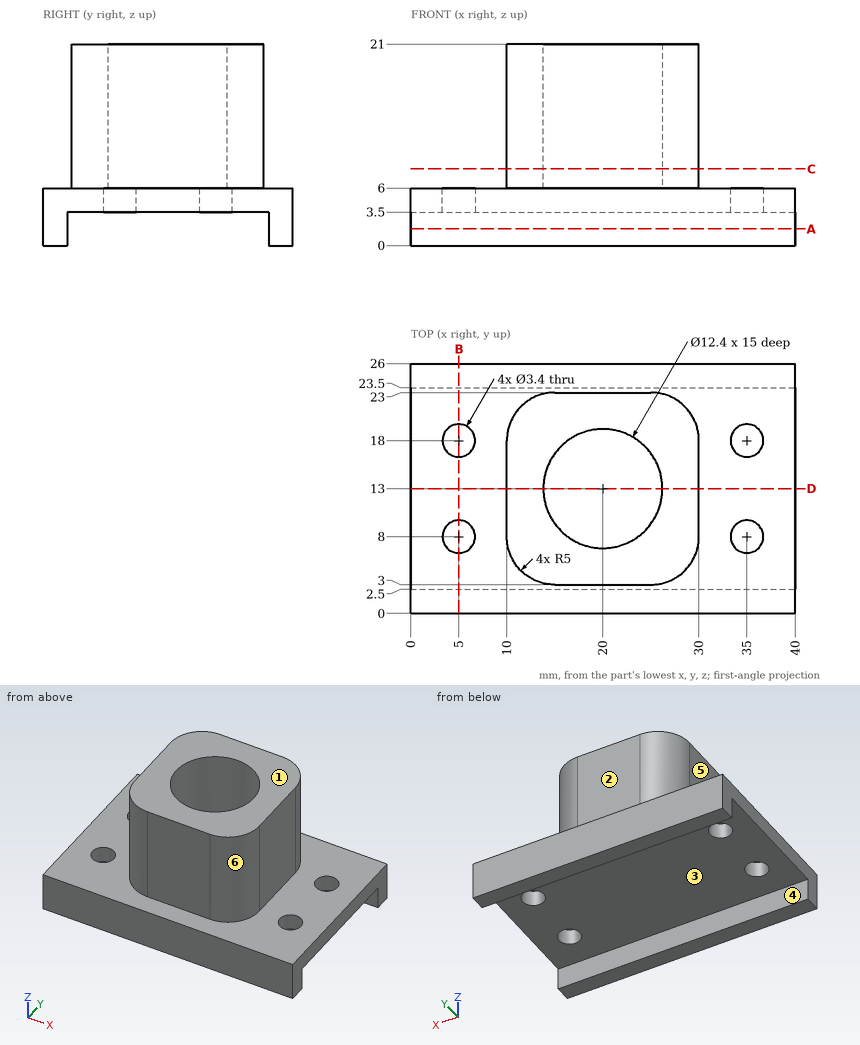
The drawing under review shows one solid part. Ordinate dimensions are in mm from its lowest x, y, z. A direction names the side the tool comes from. Round coordinates to 2 decimals unless told otherwise and drop trailing zeros. Loops run counter-clockwise (first coordinate to the right, second up) from the corner with the lowest first, then second, coordinate; pieces in that order, holes last. Notation, with made-up numbers: (28, 22) -> (58, 22) arc R23 ccw to (58, 52) -> close; hole circle Ø11 at (38, 7.25). An arc over 180 degrees is marked (long way). Answer in a Markdown table with one row per item.
1) For pin 1 Ø4.5 at (x, y) = (5, 18) entering from +Z; pin 2 Ø5.5 at (x, y) = (35, 18) entering from -Z; pin 3 Ø5 at (x, z) = (17.5, 10) entering from -Y, all flat-tipped, find the tip position at first contact; note any pin that passes through.
Taken from the geometry:
| item | result |
|---|---|
| pin 1 | stops at z = 6 |
| pin 2 | stops at z = 3.5 |
| pin 3 | stops at y = 3 |
2) Wall thickness on line 1 along Y through (x, z) = (35, 4.65); line 2 along X through (y, z) = (19, 5); line 3 along Z through (x, y) = (34.5, 6): over which ranges is each line inside the solid? List them lowest first.
Taken from the geometry:
| item | result |
|---|---|
| line 1 | y = 0 to 6.3, 9.7 to 16.3, 19.7 to 26 |
| line 2 | x = 0 to 3.63, 6.37 to 33.63, 36.37 to 40 |
| line 3 | z = 3.5 to 6 |
3) Consider section B-B, the plane x = 5. Write out the cut boundary in (y, z).
Taken from the geometry:
| item | result |
|---|---|
| outline | (0, 0) -> (2.5, 0) -> (2.5, 3.5) -> (6.3, 3.5) -> (6.3, 6) -> (0, 6) -> close; (9.7, 3.5) -> (16.3, 3.5) -> (16.3, 6) -> (9.7, 6) -> close; (19.7, 3.5) -> (23.5, 3.5) -> (23.5, 0) -> (26, 0) -> (26, 6) -> (19.7, 6) -> close |
4) Consider section D-D, the plane y = 13. Write out the cut boundary in (x, z).
Taken from the geometry:
| item | result |
|---|---|
| outline | (0, 3.5) -> (40, 3.5) -> (40, 6) -> (30, 6) -> (30, 21) -> (26.2, 21) -> (26.2, 6) -> (13.8, 6) -> (13.8, 21) -> (10, 21) -> (10, 6) -> (0, 6) -> close |
5) Consider section A-A, the plane z = 1.75. Write out the cut boundary in (x, y).
Taken from the geometry:
| item | result |
|---|---|
| outline | (0, 0) -> (40, 0) -> (40, 2.5) -> (0, 2.5) -> close; (0, 23.5) -> (40, 23.5) -> (40, 26) -> (0, 26) -> close |
6) Consider section C-C, the plane z = 8. Write out the cut boundary in (x, y), plus the area to 3 significant figures.
Taken from the geometry:
| item | result |
|---|---|
| outline | (10, 8) arc R5 ccw to (15, 3) -> (25, 3) arc R5 ccw to (30, 8) -> (30, 18) arc R5 ccw to (25, 23) -> (15, 23) arc R5 ccw to (10, 18) -> close; hole circle Ø12.4 at (20, 13) |
| area | 258 mm² |
7) Draft analysis for pull direction Y (two halves, no side actions). For the marked faces 1, 2 and 3, state which applies: pulls with the +Y half, pulls with the -Y half, needs draft (parallel to the pull), parting line crosses it, or undercut.
Taken from the geometry:
| item | result |
|---|---|
| face 1 | needs draft |
| face 2 | pulls with the +Y half |
| face 3 | undercut |
8) Tool access review of the marked faces 4, 5 and 6: name each direction out of +Z, -Z, +X, -X, +Y, -Y from which nothing blocks a thin tool from reaching the whole face with its end or side.
Taken from the geometry:
| item | result |
|---|---|
| face 4 | -Z, +X, -X |
| face 5 | +Z, -X, +Y, -Y |
| face 6 | +Z, +X, -Y |
